```python
from build123d import *

# Parameters (mm, degrees)
F0_R     = 1.6
F5_DEPTH = 5
F1_R     = 1.6
F2_W     = 70
F2_H     = 120
F2_R     = 1.6
F3_R     = 1.6
F3_R_2   = 3.5
F4_R     = 3.1
F4_R_2   = 1
F6_DEPTH = 5


with BuildPart() as f5:
    # F0 (on Top) → F5 (new body)
    with BuildSketch(Plane.XY):
        Polygon((120, 90), (-120, 90), (-120, 85), (-145, 85), (-145, 60), (-150, 60), (-150, -60), (-145, -60), (-145, -85), (-120, -85), (-120, -90), (120, -90), (120, -85), (145, -85), (145, -60), (150, -60), (150, 60), (145, 60), (145, 85), (120, 85), align=None)
        with Locations((-105, -80)):
            Circle(F0_R, mode=Mode.SUBTRACT)
        with Locations((0, -80)):
            Circle(F0_R, mode=Mode.SUBTRACT)
        with Locations((105, -80)):
            Circle(F0_R, mode=Mode.SUBTRACT)
        with Locations((-140, 0)):
            Circle(F0_R, mode=Mode.SUBTRACT)
        with Locations((-105, 80)):
            Circle(F0_R, mode=Mode.SUBTRACT)
        with Locations((140, 0)):
            Circle(F0_R, mode=Mode.SUBTRACT)
        with Locations((0, 80)):
            Circle(F0_R, mode=Mode.SUBTRACT)
        with Locations((105, 80)):
            Circle(F0_R, mode=Mode.SUBTRACT)
    extrude(amount=F5_DEPTH)

    # F1 (on face) + F2 (on face) + F3 (on face) + F4 (on face) → F6 (cut)
    with BuildSketch(Plane.XY):
        Polygon((34, 73), (-133, 73), (-133, -31), (-1, -31), (28.2220042013, -31), (29, -31), (31.171190082, -31), (34, -31), align=None)
        Polygon((28.2220042013, -31), (-1, -31), (3, -35), (25, -35), (29, -31), align=None)
        with Locations((-128, 77)):
            Circle(F1_R)
        with Locations((29, 77)):
            Circle(F1_R)
        with Locations((29, -38)):
            Circle(F1_R)
        with Locations((-128, -38)):
            Circle(F1_R)
    with BuildSketch(Plane.XY):
        with Locations((90, 13)):
            Rectangle(F2_W, F2_H)
        with Locations((131, 79)):
            Circle(F2_R)
        with Locations((115, 79)):
            Circle(F2_R)
        with Locations((131, 63)):
            Circle(F2_R)
        with Locations((65, 79)):
            Circle(F2_R)
        with Locations((49, 79)):
            Circle(F2_R)
        with Locations((49, 63)):
            Circle(F2_R)
        with Locations((49, -37)):
            Circle(F2_R)
        with Locations((49, -53)):
            Circle(F2_R)
        with Locations((65, -53)):
            Circle(F2_R)
        with Locations((115, -53)):
            Circle(F2_R)
        with Locations((131, -53)):
            Circle(F2_R)
        with Locations((131, -37)):
            Circle(F2_R)
    with BuildSketch(Plane.XY):
        with BuildLine():
            ThreePointArc((-115.4043781836, -64.8817163623), (-101.205196639, -65.2405329657), (-94, -53))
            ThreePointArc((-94, -53), (-113.715544356, -40.2198375317), (-117.3332218164, -63.4350836377))
            ThreePointArc((-117.3332218164, -63.4350836377), (-116.04, -63.72), (-115.4043781836, -64.8817163623))
        make_face()
        with BuildLine():
            ThreePointArc((-115.4043781836, -64.8817163623), (-116.04, -63.72), (-117.3332218164, -63.4350836377))
            ThreePointArc((-117.3332218164, -63.4350836377), (-116.4, -64.2), (-115.4043781836, -64.8817163623))
        make_face()
        with BuildLine():
            ThreePointArc((-115.4043781836, -64.8817163623), (-116.4, -64.2), (-117.3332218164, -63.4350836377))
            ThreePointArc((-117.3332218164, -63.4350836377), (-118.0066889027, -66.2436146723), (-115.4, -65))
            ThreePointArc((-115.4, -65), (-115.4010949205, -64.9408176812), (-115.4043781836, -64.8817163623))
        make_face()
        with Locations((-117, -39)):
            Circle(F3_R)
        with Locations((-97, -39)):
            Circle(F3_R)
        with Locations((-97, -65)):
            Circle(F3_R)
        with Locations((-83, -53)):
            Circle(F3_R_2)
        with Locations((-133, -53)):
            Circle(F3_R_2)
    with BuildSketch(Plane.XY):
        with Locations((-53, -70)):
            Circle(F4_R)
        with Locations((-53, -62.4)):
            Circle(F4_R_2)
        with Locations((-53, -50)):
            Circle(F4_R)
        with Locations((-53, -42.4)):
            Circle(F4_R_2)
        with Locations((-38, -70)):
            Circle(F4_R)
        with Locations((-38, -62.4)):
            Circle(F4_R_2)
        with Locations((-38, -50)):
            Circle(F4_R)
        with Locations((-38, -42.4)):
            Circle(F4_R_2)
        with Locations((-23, -70)):
            Circle(F4_R)
        with Locations((-23, -62.4)):
            Circle(F4_R_2)
        with Locations((-23, -50)):
            Circle(F4_R)
        with Locations((-23, -42.4)):
            Circle(F4_R_2)
    extrude(amount=F6_DEPTH, mode=Mode.SUBTRACT)


solid = f5.part
```
Check sheet for the modelled part. Datum: model origin and axes. Units: mm. Round coordinates to 2 decimals unless told otherwise and drop trailing zeros. Loops run counter-clockwise (first coordinate to the right, second up) from the corner with the lowest first, then second, coordinate; pieces in that order, holes last. Notation, with made-up numbers: (-19, 10) - (-4, 10) arc R30 cw to (-4, 33) - close; hole circle Ø6 at (12, 65). An arc over 180 degrees is marked (long way). Write item = value, one per line. Start each with the question number.
Q1. Thickness scan on L1, parallel to X at y = 19, z = 1.05; L2, parallel to Y at x = 131, z = 3.35; L3, parallel to Y at x = -38, z = 2. Record the ranges inside material, lowest first.
Q2. Section check B-B (y = 10.5). Record the boundary of the cut face in (x, z).
Q3. Section check D-D (z = 3.45). Count the separate pieces of the cut face and the enclosed holes in it, plus the area to 3 significant figures.
Q4. Depth check by flat-ended pin: P1, Ø1.5, axis at x = -148.5, z = 2, coming from the +Y side. Enter the tip coordinate at first touch or a pass-through.
Q5. Section check A-A (x = 7.5). Record the boundary of the cut face in (y, z), plus the area to 3 significant figures.
Q6. Section check C-C (x = -65.5). Record the boundary of the cut face in (y, z).
Q7. Release check for a two-part mould opening along Y. For faces 1 (the face through (-38.404, -46.926, 2.465)), 2 (the face through (-2, -39, 0)), 3 (the face through (-129.66, -51.95, 2.46)) record: pulls with the +Y half, pulls with the -Y half, needs draft (parallel to the pull), parting line crosses it, or undercut.
Derived:
q1.L1 = -150 to -133, 34 to 55, 125 to 150
q1.L2 = -85 to -54.6, -51.4 to -38.6, -35.4 to 61.4, 64.6 to 77.4, 80.6 to 85
q1.L3 = -90 to -73.1, -66.9 to -63.4, -61.4 to -53.1, -46.9 to -43.4, -41.4 to -31, 73 to 90
q2.outline = (-150, 0) - (-133, 0) - (-133, 5) - (-150, 5) - close; (34, 0) - (55, 0) - (55, 5) - (34, 5) - close; (125, 0) - (150, 0) - (150, 5) - (125, 5) - close
q3.separate_pieces = 1
q3.enclosed_holes = 44
q3.area = 25,900 mm^2
q4.P1 = 60
q5.outline = (-90, 0) - (-35, 0) - (-35, 5) - (-90, 5) - close; (73, 0) - (90, 0) - (90, 5) - (73, 5) - close
q5.area = 360 mm^2
q6.outline = (-90, 0) - (-31, 0) - (-31, 5) - (-90, 5) - close; (73, 0) - (90, 0) - (90, 5) - (73, 5) - close
q7.face_1 = undercut
q7.face_2 = needs draft
q7.face_3 = undercut
